Verification items for the finished model (mm, model axes). A direction names the side the tool comes from. Give positions to 0.01 mm unless a question says otherwise; leave off trailing zeros. Loops run counter-clockwise (first coordinate to the right, second up) from the corner with the lowest first, then second, coordinate; pieces in that order, holes last. Notation, with made-up numbers: (-16.75, 18) - (-4.75, 18) arc R13 cw to (-4.75, 25) - close; hole circle Ø7 at (21, 5). An arc over 180 degrees is marked (long way). Use one line per item in the form item = value.
```python
from build123d import *

# Parameters (mm, degrees)
BOSS_EXTRUDE1_DEPTH = 15


with BuildPart() as part:
    # Sketch1 → Boss-Extrude1 (new body)
    with BuildSketch(Plane(origin=(0, 0, 0), x_dir=(0, 0, -1), z_dir=(1, 0, 0))):
        with BuildLine():
            Line((0, 24.35), (1465, 24.35))
            ThreePointArc((1465, 24.35), (1489.35, 0), (1465, -24.35))
            Line((1465, -24.35), (0, -24.35))
            ThreePointArc((0, -24.35), (-24.35, 0), (0, 24.35))
        make_face()
        with BuildLine():
            Line((0, 23.4), (1465, 23.4))
            ThreePointArc((1465, 23.4), (1488.4, 0), (1465, -23.4))
            Line((1465, -23.4), (0, -23.4))
            ThreePointArc((0, -23.4), (-23.4, 0), (0, 23.4))
        make_face(mode=Mode.SUBTRACT)
    extrude(amount=-BOSS_EXTRUDE1_DEPTH)


solid = part.part
```
1. Section check B-B, the plane y = 9. Record the cut outline in (x, z).
Result set:
outline = (-15, -1487.63) - (0, -1487.63) - (0, -1486.6) - (-15, -1486.6) - close; (-15, 21.6) - (0, 21.6) - (0, 22.63) - (-15, 22.63) - close
2. Draft check along Z on faces 1 (the flat face through (0, 24, -736)), 2 (the cylindrical face through (-7.395, 0.515, -1488.394)), 3 (the cylindrical face through (-7.395, 0.535, -1489.344)). Enter one of: released by +Z, released by -Z, zero draft, split by the parting line, or undercut.
Result set:
face_1 = zero draft
face_2 = undercut
face_3 = released by -Z
3. Tool access check on faces 4 (the cylindrical face through (-7.395, -0.535, 24.344)), 5 (the cylindrical face through (-7.395, -0.515, 23.394)). Record the directions out of +Z, -Z, +X, -X, +Y, -Y that give a thin tool (end or side, any length) a straight path to the whole face; none if there is none.
Result set:
face_4 = +Z, +X, -X
face_5 = +X, -X
4. Depth check by flat-ended pin: pin 1 Ø2 at (x, y) = (-12, 15.5) entering from -Z. Enter the tip coordinate at first touch or a pass-through.
Result set:
pin_1 = -1484.56
5. Section check C-C, the plane x = -8.25. Record the cut outline in (y, z), then the cut area to 3 significant figures.
Result set:
outline = (-24.35, -1465) arc R24.35 ccw to (24.35, -1465) - (24.35, 0) arc R24.35 ccw to (-24.35, 0) - close; hole (-23.4, -1465) arc R23.4 ccw to (23.4, -1465) - (23.4, 0) arc R23.4 ccw to (-23.4, 0) - close
area = 2,930 mm²
6. Section check A-A, the plane z = -724. Record the cut outline in (x, y).
Result set:
outline = (-15, -24.35) - (0, -24.35) - (0, -23.4) - (-15, -23.4) - close; (-15, 23.4) - (0, 23.4) - (0, 24.35) - (-15, 24.35) - close
7. Scan lines: probe 1 along Y at (x, z) = (-8.25, -1313); probe 2 along Z at (x, y) = (-3.75, -2.5). Record each from-to range of solid material in increasing order.
Result set:
probe_1 = -24.35 to -23.4, 23.4 to 24.35
probe_2 = -1489.22 to -1488.27, 23.27 to 24.22
